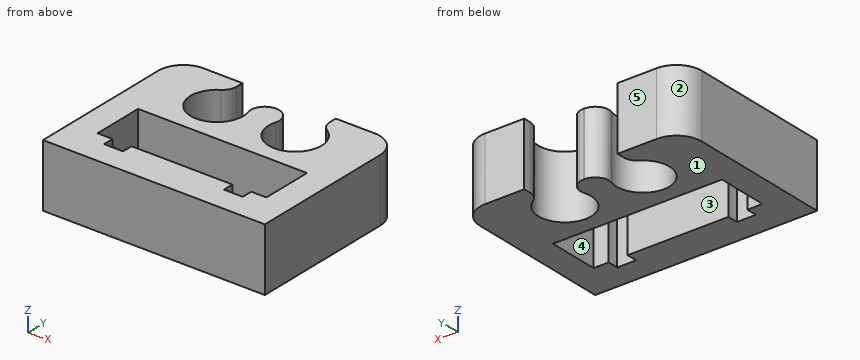
from build123d import *

# Parameters (mm, degrees)
SKETCH1_W           = 17.6
SKETCH1_H           = 13.5
BOSS_EXTRUDE1_DEPTH = 5
SKETCH2_W           = 1.5
SKETCH2_H           = 0.85
SKETCH2_W_2         = 13.4
SKETCH2_H_2         = 4.05
CUT_EXTRUDE2_DEPTH  = 5
SKETCH3_R           = 2.1
SKETCH3_W           = 7.4
SKETCH3_H           = 1.3
CUT_EXTRUDE3_DEPTH  = 5
FILLET1_R           = 1.1
FILLET2_R           = 2


with BuildPart() as part:
    # Sketch1 → Boss-Extrude1 (new body)
    with BuildSketch(Plane.XY):
        with Locations((8.8, 6.75)):
            Rectangle(SKETCH1_W, SKETCH1_H)
    extrude(amount=BOSS_EXTRUDE1_DEPTH)

    # Sketch2 → Cut-Extrude2 (cut)
    with BuildSketch(Plane.XY.offset(5)):
        with Locations((13.55, 2.375)):
            Rectangle(SKETCH2_W, SKETCH2_H)
        with Locations((8.8, 4.825)):
            Rectangle(SKETCH2_W_2, SKETCH2_H_2)
        with Locations((4.05, 2.375)):
            Rectangle(SKETCH2_W, SKETCH2_H)
    extrude(amount=-CUT_EXTRUDE2_DEPTH, mode=Mode.SUBTRACT)

    # Sketch3 → Cut-Extrude3 (cut)
    with BuildSketch(Plane.XY.offset(5)):
        with Locations((5.7, 10.2)):
            Circle(SKETCH3_R)
        with Locations((11.9, 10.2)):
            Circle(SKETCH3_R)
        with Locations((8.8, 12.85)):
            Rectangle(SKETCH3_W, SKETCH3_H)
    extrude(amount=-CUT_EXTRUDE3_DEPTH, mode=Mode.SUBTRACT)

    # Fillet1
    fillet1_edges = [part.edges().sort_by_distance(p)[0] for p in [
        (12.5, 12.21246118, 2.5),
        (5.1, 12.21246118, 2.5),
        (6.340312424, 12.2, 2.5),
        (11.259687576, 12.2, 2.5),
    ]]
    fillet(fillet1_edges, radius=FILLET1_R)

    # Fillet2
    fillet2_edges = [part.edges().sort_by_distance(p)[0] for p in [
        (0, 13.5, 2.5),
        (17.6, 13.5, 2.5),
    ]]
    fillet(fillet2_edges, radius=FILLET2_R)


solid = part.part
The model under review builds one solid part; all positions refer to its coordinate system, in mm. Face numbers are marked on the shaded views. A direction names the side the tool comes from. Coordinates: 2 decimals unless noted, no trailing zeros. Write each loop counter-clockwise with the first axis right and the second up, starting at its lowest first coordinate (ties: lowest second). Pieces come first, ordered by that corner, then holes. Notation, with made-up numbers: (-19.75, 35) - (19.25, 35) arc R18 ccw to (19.25, 40) - close; hole circle Ø10 at (24.5, 66). An arc over 180 degrees is marked (long way). Answer as a JSON object with one key per item and string values. Group by question number.
1. Add section C-C (y = 2.25). Give the boundary of the cut face in (x, z).
2. Mouldability with a two-part tool opening along Y and no side actions: class the marked faces 1, 2 and 3 as pulls with the +Y half, pulls with the -Y half, needs draft (parallel to the pull), parting line crosses it, or undercut.
3. Add section D-D (z = 1.3). Give the boundary of the cut face in (x, y), plus the area to 3 significant figures.
4. To check wall thickness, follow probe 1 along X at (y, z) = (10.2, 3.1); probe 2 along X at (y, z) = (11.75, 2.95); probe 3 along Y at (x, z) = (11.9, 2.15). State the ranges of each line that lie inside material, in increasing order.
5. Add section A-A (y = 4.5). Give the boundary of the cut face in (x, z).
6. Add section B-B (x = 11.9). Give the boundary of the cut face in (y, z).
7. Clearance check with a flat-ended pin moving along its axis: pin 1 Ø1 at (x, z) = (6, 1.5) entering from +Y. State where the tip first meets the part, or that it passes through.
8. Machinability: for the marked faces 4 and 5, which of the approach directions +Z, -Z, +X, -X, +Y, -Y give a long, thin tool a straight path to every point of the face, cutting with its end or side? Answer none if there is none.
Findings:
{
 "1": {"outline": "(0, 0) - (3.3, 0) - (3.3, 5) - (0, 5) - close; (4.8, 0) - (12.8, 0) - (12.8, 5) - (4.8, 5) - close; (14.3, 0) - (17.6, 0) - (17.6, 5) - (14.3, 5) - close"},
 "2": {"face 1": "needs draft", "face 2": "pulls with the +Y half", "face 3": "undercut"},
 "3": {"outline": "(0, 0) - (17.6, 0) - (17.6, 11.5) arc R2 ccw to (15.6, 13.5) - (12.5, 13.5) - (12.5, 12.91) arc R1.1 ccw to (13.02, 11.98) arc R2.1 cw (long way) to (9.88, 10.79) arc R1.1 ccw to (8.83, 12.2) - (8.77, 12.2) arc R1.1 ccw to (7.72, 10.79) arc R2.1 cw (long way) to (4.58, 11.98) arc R1.1 ccw to (5.1, 12.91) - (5.1, 13.5) - (2, 13.5) arc R2 ccw to (0, 11.5) - close; hole (2.1, 2.8) - (3.3, 2.8) - (3.3, 1.95) - (4.8, 1.95) - (4.8, 2.8) - (12.8, 2.8) - (12.8, 1.95) - (14.3, 1.95) - (14.3, 2.8) - (15.5, 2.8) - (15.5, 6.85) - (2.1, 6.85) - close", "area": "140 mm²"},
 "4": {"probe 1": "0 to 3.6, 7.8 to 9.8, 14 to 17.6", "probe 2": "0.02 to 4.28, 7.88 to 9.72, 13.32 to 17.58", "probe 3": "0 to 2.8, 6.85 to 8.1"},
 "5": {"outline": "(0, 0) - (2.1, 0) - (2.1, 5) - (0, 5) - close; (15.5, 0) - (17.6, 0) - (17.6, 5) - (15.5, 5) - close"},
 "6": {"outline": "(0, 0) - (2.8, 0) - (2.8, 5) - (0, 5) - close; (6.85, 0) - (8.1, 0) - (8.1, 5) - (6.85, 5) - close"},
 "7": {"pin 1": "y = 8.26"},
 "8": {"face 4": "+Z, -Z", "face 5": "+Z, -Z, +X, -X, +Y"}
}
